```python
from build123d import *

# Parameters (mm, degrees)
ESQUISSE1_W             = 82.55
ESQUISSE1_H             = 914.4
BOSS_EXTRU_1_DEPTH      = 15.875
ENL_V_MAT_EXTRU_1_DEPTH = 916.468733082


with BuildPart() as part:
    # Esquisse1 → Boss.-Extru.1 (new body)
    with BuildSketch(Plane(origin=(0, 0, 0), x_dir=(0, 0, -1), z_dir=(1, 0, 0))):
        Rectangle(ESQUISSE1_W, ESQUISSE1_H)
    extrude(amount=BOSS_EXTRU_1_DEPTH)

    # Esquisse3 → Enlèv. mat.-Extru.1 (cut, through all)
    with BuildSketch(Plane(origin=(0, 457.2, 0), x_dir=(1, 0, 0), z_dir=(0, 1, 0))):
        Polygon((12.7, 41.275), (38.1, 41.275), (38.1, -41.275), (12.7, -41.275), (12.7, -13.5), (19.05, -13.5), (19.05, 13.5), (12.7, 13.5), align=None)
    extrude(amount=-ENL_V_MAT_EXTRU_1_DEPTH, mode=Mode.SUBTRACT)


solid = part.part
```
Work out the finished part from the listing and answer in its coordinate system (mm). A direction names the side the tool comes from. Coordinates: 2 decimals unless noted, no trailing zeros. Write each loop counter-clockwise with the first axis right and the second up, starting at its lowest first coordinate (ties: lowest second). Pieces come first, ordered by that corner, then holes.
Q1. A cutting plane is placed at B-B, the plane z = 23.5. Give the vertices of the cut face in (x, y).
Q2. Determine the mould class of faces 1 (the face through (15.875, 6, 0)), 2 (the face through (6, -457.2, 1)), 3 (the face through (0, 6, 1)) for opening direction X: released by +X, released by -X, zero draft, split by the parting line, or undercut.
Q3. Each of these flat-tipped pins is pushed along its axis until it touches: pin 1 Ø1 at (x, y) = (15, -14) entering from -Z; pin 2 Ø22 at (y, z) = (22, -29.5) entering from +X; pin 3 Ø2.5 at (x, y) = (14, -143) entering from +Z. Where does it stop, or does it pass through?
Q4. Find the intervals of material crossed by line 1 (X direction, y = 317, z = 32); line 2 (Z direction, x = 14, y = 279.5), in increasing order.
Q5. Which of the six approach directions +Z, -Z, +X, -X, +Y, -Y give full straight-line access (tool end or side, diameter ignored) to faces 4 (the face through (12.7, 6, 28)), 5 (the face through (6, 457.2, 1)), 6 (the face through (12.7, 6, -27))?
Q6. A cutting plane is placed at A-A, the plane y = 84. Give the vertices of the cut face in (x, z) (3 decimals), then the cut area to 3 significant figures.
Findings below:
1. outline: (0, -457.2) - (12.7, -457.2) - (12.7, 457.2) - (0, 457.2) - close
2. face 1: released by +X
2. face 2: zero draft
2. face 3: released by -X
3. pin 1: stops at z = -13.5
3. pin 2: stops at x = 12.7
3. pin 3: stops at z = 13.5
4. line 1: x = 0 to 12.7
4. line 2: z = -13.5 to 13.5
5. face 4: +Z, +X, +Y, -Y
5. face 5: +Z, -Z, +X, -X, +Y
5. face 6: -Z, +X, +Y, -Y
6. outline: (0, -41.275) - (12.7, -41.275) - (12.7, -13.5) - (15.875, -13.5) - (15.875, 13.5) - (12.7, 13.5) - (12.7, 41.275) - (0, 41.275) - close
6. area: 1,130 mm2
